from build123d import *

# Parameters (mm, degrees)
SKETCH1_W           = 38.1
SKETCH1_H           = 101.6
SKETCH1_R           = 10.85
BOSS_EXTRUDE1_DEPTH = 6.35
FILLET1_R           = 5
FILLET2_R           = 5
FILLET3_R           = 5
FILLET4_R           = 5
CUT_EXTRUDE1_REACH  = 180.93
SKETCH2_R           = 4.445


with BuildPart() as part:
    # Sketch1 → Boss-Extrude1 (new body)
    with BuildSketch(Plane.XY):
        with Locations((0, -127)):
            Rectangle(SKETCH1_W, SKETCH1_H)
        with Locations((-1.778, -135.128)):
            Circle(SKETCH1_R, mode=Mode.SUBTRACT)
    extrude(amount=BOSS_EXTRUDE1_DEPTH)

    # Fillet1
    fillet1_edges = [part.edges().sort_by_distance(p)[0] for p in [
        (-19.05, -76.2, 3.175),
    ]]
    fillet(fillet1_edges, radius=FILLET1_R)

    # Fillet2
    fillet2_edges = [part.edges().sort_by_distance(p)[0] for p in [
        (19.05, -76.2, 3.175),
    ]]
    fillet(fillet2_edges, radius=FILLET2_R)

    # Fillet3
    fillet3_edges = [part.edges().sort_by_distance(p)[0] for p in [
        (19.05, -177.8, 3.175),
    ]]
    fillet(fillet3_edges, radius=FILLET3_R)

    # Fillet4
    fillet4_edges = [part.edges().sort_by_distance(p)[0] for p in [
        (-19.05, -177.8, 3.175),
    ]]
    fillet(fillet4_edges, radius=FILLET4_R)

    # Sketch2 → Cut-Extrude1 (cut, up to next)
    with BuildSketch(Plane.XY.offset(6.35), mode=Mode.PRIVATE) as cut_extrude1_sk1:
        with Locations((0, -99.788381621)):
            Circle(SKETCH2_R)
    cut_extrude1_tool1 = extrude(cut_extrude1_sk1.sketch, amount=-CUT_EXTRUDE1_REACH, mode=Mode.PRIVATE) & part.part
    # Sketch2 → Cut-Extrude1 (cut, up to next)
    with BuildSketch(Plane.XY.offset(6.35), mode=Mode.PRIVATE) as cut_extrude1_sk2:
        with Locations((0, -162.625541616)):
            Circle(SKETCH2_R)
    cut_extrude1_tool2 = extrude(cut_extrude1_sk2.sketch, amount=-CUT_EXTRUDE1_REACH, mode=Mode.PRIVATE) & part.part
    add(cut_extrude1_tool1.solids().sort_by_distance((0, -99.788382, 6.35))[0], mode=Mode.SUBTRACT)
    add(cut_extrude1_tool2.solids().sort_by_distance((0, -162.625542, 6.35))[0], mode=Mode.SUBTRACT)


solid = part.part
Here's how the part is built. I have some questions about the finished solid (model axes, mm). Give positions to 0.01 mm unless a question says otherwise; leave off trailing zeros. Order: outer loops, then holes, each group sorted by start corner. A loop starts at its lowest first (then second) coordinate and runs counter-clockwise, first axis right, second up. Notation, with made-up numbers: (-2.75, 41) -> (19.25, 41) arc R26 ccw to (19.25, 80) -> close; hole circle Ø10 at (70, 46.25). An arc over 180 degrees is marked (long way). Use a Markdown table: item, result. Add a question column.
Item 1: Imagine slicing it at D-D on z = 3.75. Please give me the cut outline in (x, y) (3 decimals).
Item 2: I need wall thicknesses on line 1 (Y direction, x = 0, z = 3); line 2 (Y direction, x = 1.5, z = 2.25); line 3 (Y direction, x = 15, z = 4.75). Which ranges of each line are inside material? Lowest first, please.
Item 3: Imagine slicing it at C-C on x = 7.5. Please give me the cut outline in (y, z), plus the area to 3 significant figures.
Item 4: If we mould it in two halves opening along Y, with no side actions, what happens to faces 1 (the face through (17.55, -77.63, 3.22)), 2 (the face through (-3.19, -124.37, 3.13)), 3 (the face through (8, -126, 0)), 4 (the face through (17.62, -176.3, 3.22))? For each: pulls with the +Y half, pulls with the -Y half, needs draft (parallel to the pull), parting line crosses it, or undercut.
Item 5: Imagine slicing it at B-B on y = -164.5. Please give me the cut outline in (x, z).
Item 6: Will this pin go through, and if not, where does the flat tip stop? pin 1 (7 mm diameter, centred on x = 0, y = -99.79, fed in from -Z).
Item 7: Imagine slicing it at A-A on x = 0. Please give me the cut outline in (y, z), plus the area to 3 significant figures.
Data:
| question | item | result |
|---|---|---|
| 1 | outline | (-19.05, -172.8) arc R5 ccw to (-14.05, -177.8) -> (14.05, -177.8) arc R5 ccw to (19.05, -172.8) -> (19.05, -81.2) arc R5 ccw to (14.05, -76.2) -> (-14.05, -76.2) arc R5 ccw to (-19.05, -81.2) -> close; hole circle Ø21.7 at (-1.778, -135.128); hole circle Ø8.89 at (0, -162.626); hole circle Ø8.89 at (0, -99.788) |
| 2 | line 1 | y = -177.8 to -167.07, -158.18 to -145.83, -124.42 to -104.23, -95.34 to -76.2 |
| 2 | line 2 | y = -177.8 to -166.81, -158.44 to -145.47, -124.79 to -103.97, -95.6 to -76.2 |
| 2 | line 3 | y = -177.71 to -76.29 |
| 3 | outline | (-177.8, 0) -> (-140.75, 0) -> (-140.75, 6.35) -> (-177.8, 6.35) -> close; (-129.5, 0) -> (-76.2, 0) -> (-76.2, 6.35) -> (-129.5, 6.35) -> close |
| 3 | area | 574 mm² |
| 4 | face 1 | pulls with the +Y half |
| 4 | face 2 | undercut |
| 4 | face 3 | needs draft |
| 4 | face 4 | pulls with the -Y half |
| 5 | outline | (-19.05, 0) -> (-4.03, 0) -> (-4.03, 6.35) -> (-19.05, 6.35) -> close; (4.03, 0) -> (19.05, 0) -> (19.05, 6.35) -> (4.03, 6.35) -> close |
| 6 | pin 1 | passes through |
| 7 | outline | (-177.8, 0) -> (-167.07, 0) -> (-167.07, 6.35) -> (-177.8, 6.35) -> close; (-158.18, 0) -> (-145.83, 0) -> (-145.83, 6.35) -> (-158.18, 6.35) -> close; (-124.42, 0) -> (-104.23, 0) -> (-104.23, 6.35) -> (-124.42, 6.35) -> close; (-95.34, 0) -> (-76.2, 0) -> (-76.2, 6.35) -> (-95.34, 6.35) -> close |
| 7 | area | 396 mm² |
